Read the model definition and answer for the solid it produces. Units are mm, in the model's axes. Coordinates: 2 decimals unless noted, no trailing zeros. Order: outer loops, then holes, each group sorted by start corner. A loop starts at its lowest first (then second) coordinate and runs counter-clockwise, first axis right, second up. Notation, with made-up numbers: (70.5, 12.25) - (118.5, 12.25) arc R12 cw to (118.5, 24.25) - close; hole circle Ø4 at (-39, 56). An arc over 180 degrees is marked (long way). Use one line per item in the form item = value.
```python
from build123d import *

# Parameters (mm, degrees)
F2_R     = 5
F2_R_2   = 4.7874181829
F3_DEPTH = 25
F4_DEPTH = 18
F2_R_3   = 13
F5_DEPTH = 6
F6_SIZE  = 3


# Not quite as in the source:
# - a feature names something its author has since deleted; it is built from what else it names


with BuildPart() as f1:
    # F0 (on Front) → F1 (revolve)
    with BuildSketch(Plane.XZ):
        with BuildLine():
            Line((0, 27), (0, 0))
            Line((0, 0), (15, 0))
            Line((15, 0), (12, 15))
            ThreePointArc((12, 15), (8.4852813742, 23.4852813742), (0, 27))
        make_face()
    revolve(axis=Axis((0, 0, 13.5), (0, 0, -1)))

    # F2 (on face) → F3 (cut)
    with BuildSketch(Plane(origin=(0, 0, 0), x_dir=(1, 0, 0), z_dir=(0, 0, -1))):
        Circle(F2_R)
        Circle(F2_R_2, mode=Mode.SUBTRACT)
        Circle(F2_R_2)
    extrude(amount=-F3_DEPTH, mode=Mode.SUBTRACT)

    # F2 (on face) → F4 (cut)
    with BuildSketch(Plane(origin=(0, 0, 0), x_dir=(1, 0, 0), z_dir=(0, 0, -1))):
        Polygon((9, -3.7279220614), (9, 3.7279220614), (3.7279220614, 9), (-3.7279220614, 9), (-9, 3.7279220614), (-9, -3.7279220614), (-3.7279220614, -9), (3.7279220614, -9), align=None)
        Circle(F2_R, mode=Mode.SUBTRACT)
    extrude(amount=-F4_DEPTH, mode=Mode.SUBTRACT)

    # F2 (on face) → F5 (cut)
    with BuildSketch(Plane(origin=(0, 0, 0), x_dir=(1, 0, 0), z_dir=(0, 0, -1))):
        Circle(F2_R_3)
        Polygon((3.7279220614, 9), (9, 3.7279220614), (9, -3.7279220614), (3.7279220614, -9), (-3.7279220614, -9), (-9, -3.7279220614), (-9, 3.7279220614), (-3.7279220614, 9), align=None, mode=Mode.SUBTRACT)
    extrude(amount=-F5_DEPTH, mode=Mode.SUBTRACT)

    # F6
    f6_edges = [f1.edges().sort_by_distance(p)[0] for p in [
        (-5, 0, 25),
        (-13, 0, 6),
        (0, 9, 18),
        (6.363961, 6.363961, 18),
        (9, 0, 18),
        (-6.363961, 6.363961, 18),
        (-9, 0, 18),
        (-6.363961, -6.363961, 18),
        (0, -9, 18),
        (6.363961, -6.363961, 18),
    ]]
    chamfer(f6_edges, length=F6_SIZE)


solid = f1.part
```
(1) Section B-B, the plane y = 0 is taken. Write down the section's boundary in (x, z), then the cut area to 3 significant figures.
Answer list:
outline = (-15, 0) - (-13, 0) - (-13, 3) - (-10, 6) - (-9, 6) - (-9, 15) - (-6, 18) - (-5, 18) - (-5, 22) - (-2, 25) - (2, 25) - (5, 22) - (5, 18) - (6, 18) - (9, 15) - (9, 6) - (10, 6) - (13, 3) - (13, 0) - (15, 0) - (12, 15) arc R12 ccw to (-12, 15) - close
area = 216 mm2
(2) The mould has two halves that part along X. Classify faces 1 (the flat face through (-6.33, -6.4, 10.44)), 2 (the conical face through (-2.777, 12.508, 10.938)), 3 (the flat face through (0.1, -13.4, 0)): +X half, -X half, draft (parallel to the pull), parting line (faces both ways), or undercut.
Answer list:
face_1 = undercut
face_2 = parting line
face_3 = draft
(3) Straight lines are drawn through the part: L1, parallel to Y at x = -0.75, z = 22.5; L2, parallel to X at y = -4, z = 19.25; L3, parallel to Z at x = 0, y = 0.5. For each, find the intervals that lie inside material, in ascending order.
Answer list:
L1 = -9.34 to -4.44, 4.44 to 9.34
L2 = -10.49 to -3, 3 to 10.49
L3 = 25 to 26.99
(4) Given pin 1 Ø3.5 at (y, z) = (0, 12) entering from -X; pin 2 Ø4.5 at (x, y) = (-0.5, -1) entering from -Z; pin 3 Ø2 at (y, z) = (1.5, 4.5) entering from +X, each flat-ended and moving along its own axis, determine where each tip first touches the part or whether it passes through.
Answer list:
pin_1 = -12.95
pin_2 = 23.63
pin_3 = 14.24
(5) Section A-A, the plane z = 10 is taken. Write down the section's boundary in (x, y), then the cut area to 3 significant figures.
Answer list:
outline = circle Ø26 at (0, 0); hole (-9, -3.73) - (-3.73, -9) - (3.73, -9) - (9, -3.73) - (9, 3.73) - (3.73, 9) - (-3.73, 9) - (-9, 3.73) - close
area = 263 mm2
(6) Section D-D, the plane z = 4.75 is taken. Write down the section's boundary in (x, y), then the cut area to 3 significant figures.
Answer list:
outline = circle Ø28.1 at (0, 0); hole circle Ø22.5 at (0, 0)
area = 223 mm2
